from build123d import *

# Parameters (mm, degrees)
SKETCH1_R           = 50
SKETCH1_R_2         = 45
SKETCH1_R_3         = 29.325
SKETCH1_R_4         = 27.5
SKETCH1_R_5         = 22.5
SKETCH1_R_6         = 22
BOSS_EXTRUDE1_DEPTH = 5
SKETCH1_3_R         = 29.325
SKETCH1_3_R_2       = 27.5
BOSS_EXTRUDE2_DEPTH = 18
SKETCH2_R           = 29.75
SKETCH2_R_2         = 29.325
BOSS_EXTRUDE3_DEPTH = 2.3
SKETCH3_R           = 27.5
SKETCH3_R_2         = 25
BOSS_EXTRUDE4_DEPTH = 2
CUT_EXTRUDE1_START  = -4
SKETCH4_R           = 25
SKETCH4_R_2         = 22
CUT_EXTRUDE1_DEPTH  = 4


with BuildPart() as part:
    # Sketch1 → Boss-Extrude1 (new body)
    # profile 1 of 5: a face of its own
    with BuildSketch(Plane.XY):
        Circle(SKETCH1_R)
        Circle(SKETCH1_R_2, mode=Mode.SUBTRACT)
    # profile 2 of 5: a face of its own
    with BuildSketch(Plane.XY):
        Circle(SKETCH1_R_2)
        Circle(SKETCH1_R_3, mode=Mode.SUBTRACT)
    # profile 3 of 5: a face of its own
    with BuildSketch(Plane.XY):
        Circle(SKETCH1_R_3)
        Circle(SKETCH1_R_4, mode=Mode.SUBTRACT)
    # profile 4 of 5: a face of its own
    with BuildSketch(Plane.XY):
        Circle(SKETCH1_R_4)
        Circle(SKETCH1_R_5, mode=Mode.SUBTRACT)
    # profile 5 of 5: a face of its own
    with BuildSketch(Plane.XY):
        Circle(SKETCH1_R_5)
        Circle(SKETCH1_R_6, mode=Mode.SUBTRACT)
    extrude(amount=BOSS_EXTRUDE1_DEPTH)

    # Sketch1_3 → Boss-Extrude2 (add)
    with BuildSketch(Plane.XY):
        Circle(SKETCH1_3_R)
        Circle(SKETCH1_3_R_2, mode=Mode.SUBTRACT)
    extrude(amount=BOSS_EXTRUDE2_DEPTH)

    # Sketch2 → Boss-Extrude3 (add)
    with BuildSketch(Plane.XY.offset(5)):
        Circle(SKETCH2_R)
        Circle(SKETCH2_R_2, mode=Mode.SUBTRACT)
    extrude(amount=BOSS_EXTRUDE3_DEPTH)

    # Sketch3 → Boss-Extrude4 (add)
    with BuildSketch(Plane.XY.offset(5)):
        Circle(SKETCH3_R)
        Circle(SKETCH3_R_2, mode=Mode.SUBTRACT)
    extrude(amount=BOSS_EXTRUDE4_DEPTH)

    # Sketch4 → Cut-Extrude1 (cut)
    with BuildSketch(Plane.XY.offset(5).offset(CUT_EXTRUDE1_START)):
        Circle(SKETCH4_R)
        Circle(SKETCH4_R_2, mode=Mode.SUBTRACT)
    extrude(amount=CUT_EXTRUDE1_DEPTH, mode=Mode.SUBTRACT)


solid = part.part
Source: CAD feature listing. Evaluate the final solid. Frame: model axes, mm. A direction names the side the tool comes from. Give positions to 0.01 mm unless a question says otherwise; leave off trailing zeros. Order: outer loops, then holes, each group sorted by start corner. A loop starts at its lowest first (then second) coordinate and runs counter-clockwise, first axis right, second up. Notation, with made-up numbers: (34.25, 51) -> (54.25, 51) arc R19 ccw to (54.25, 63) -> close; hole circle Ø4 at (86.5, -1.75). An arc over 180 degrees is marked (long way). Use a Markdown table: item, result.
1) Mould query, pull axis X, two halves, no side actions, for faces 3 (the cylindrical face through (23.846, 7.509, 3.958)), 4 (the cylindrical face through (15.993, 25.085, 6.134)), 5 (the flat face through (-13.4, -26.3, 7.3)). Classes: +X half, -X half, draft (parallel to the pull), parting line (faces both ways), or undercut.
Answer list:
| item | result |
|---|---|
| face 3 | undercut |
| face 4 | parting line |
| face 5 | draft |
2) Reachability of faces 1 (the flat face through (1.7, -22.1, 1)), 2 (the cylindrical face through (-4.769, -21.477, 0.493)) from +Z, -Z, +X, -X, +Y, -Y: full face, straight path, thin tool, end or side. Return the list, or none.
Answer list:
| item | result |
|---|---|
| face 1 | +Z |
| face 2 | +Z, -Z |
3) Section query A-A, the plane y = 0. Return the cut outline in (x, z) (3 decimals), then the cut area to 3 significant figures.
Answer list:
| item | result |
|---|---|
| outline | (-50, 0) -> (-22, 0) -> (-22, 1) -> (-25, 1) -> (-25, 7) -> (-27.5, 7) -> (-27.5, 18) -> (-29.325, 18) -> (-29.325, 7.3) -> (-29.75, 7.3) -> (-29.75, 5) -> (-50, 5) -> close; (22, 0) -> (50, 0) -> (50, 5) -> (29.75, 5) -> (29.75, 7.3) -> (29.325, 7.3) -> (29.325, 18) -> (27.5, 18) -> (27.5, 7) -> (25, 7) -> (25, 1) -> (22, 1) -> close |
| area | 315 mm² |
4) Section query D-D, the plane y = 40. Return the cut outline in (x, z).
Answer list:
| item | result |
|---|---|
| outline | (-30, 0) -> (30, 0) -> (30, 5) -> (-30, 5) -> close |
5) Contact query for flat-ended pins moving along their axis: P1, Ø6, axis at y = 5.5, z = 15, coming from the -X side; P2, Ø4, axis at y = 24.5, z = 12, coming from the -X side; P3, Ø3, axis at x = -8, z = 7, coming from the -Y side; P4, Ø1, axis at x = -16.5, y = -12, coming from the +Z side. Output: stop coordinate, or through.
Answer list:
| item | result |
|---|---|
| P1 | x = -29.22 |
| P2 | x = -18.81 |
| P3 | y = -29.03 |
| P4 | through |
6) Section query C-C, the plane z = 10.25. Return the cut outline in (x, y) (3 decimals), then the cut area to 3 significant figures.
Answer list:
| item | result |
|---|---|
| outline | circle Ø58.65 at (0, 0); hole circle Ø55 at (0, 0) |
| area | 326 mm² |
7) Ray query, line 1 along X through (y, z) = (-0.5, 10.5); line 2 along Y through (x, z) = (0, 4.9); line 3 along Y through (x, z) = (0, 0.4). Return the intervals inside material, ascending. Write a range as [from, to].
Answer list:
| item | result |
|---|---|
| line 1 | [-29.32, -27.5], [27.5, 29.32] |
| line 2 | [-50, -25], [25, 50] |
| line 3 | [-50, -22], [22, 50] |
